Check sheet for the drawn part. Datum: minimum x, y, z corner. Units: mm. A direction names the side the tool comes from. Coordinates: 2 decimals unless noted, no trailing zeros. Loops run counter-clockwise (first coordinate to the right, second up) from the corner with the lowest first, then second, coordinate; pieces in that order, holes last.
Q1. Sectioned sample at A-A (z = 0.7). Count the separate pieces of the cut face and the enclosed holes in it, then the cut area to 3 significant figures.
Q2. Sectioned sample at C-C (y = 3). Enter the section's corners in (x, z), then the cut area to 3 significant figures.
Q3. Go/stop test with a flat-tipped pin: P1, Ø1, axis at x = 1.5, z = 5, coming from the -Y side. Record where the tip stops, or that it passes through.
Q4. Sectioned sample at D-D (y = 6.25). Enter the section's corners in (x, z).
Q5. Sectioned sample at B-B (x = 5). Enter the section's corners in (y, z).
Q6. Mould release check, pull along Z, two halves, no side actions. Record for the marked faces 3, 4 and 5: +Z half, -Z half, draft (parallel to the pull), parting line (faces both ways), or undercut.
Q7. Material ranges on probe 1 along Y at (x, z) = (5, 4.5); probe 2 along X at (y, z) = (7, 1.95); probe 3 along Y at (x, z) = (5, 0.6), recorded low to high.
Q8. Access from +Z, -Z, +X, -X, +Y, -Y to the whole of each face (thin tool, end or side, straight path). Record for the marked faces 1 and 2.
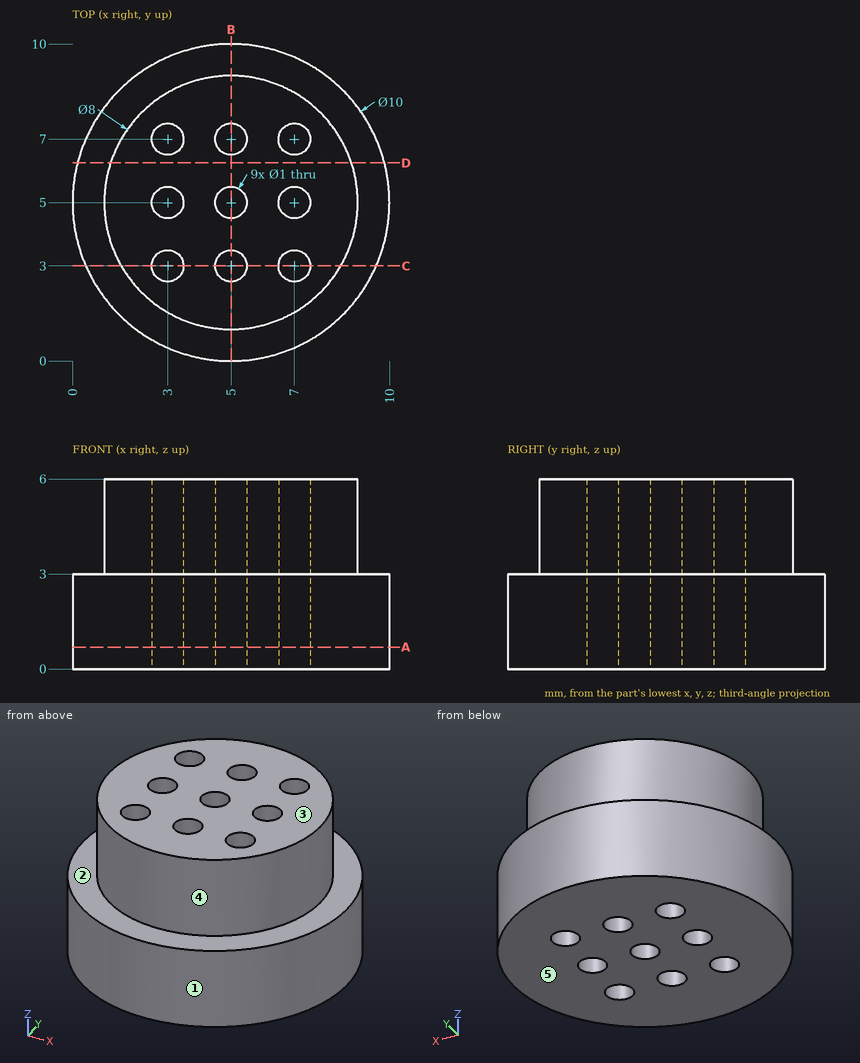
Geometry check:
1. separate pieces: 1
1. enclosed holes: 9
1. area: 71.5 mm2
2. outline: (0.42, 0) - (2.5, 0) - (2.5, 6) - (1.54, 6) - (1.54, 3) - (0.42, 3) - close; (3.5, 0) - (4.5, 0) - (4.5, 6) - (3.5, 6) - close; (5.5, 0) - (6.5, 0) - (6.5, 6) - (5.5, 6) - close; (7.5, 0) - (9.58, 0) - (9.58, 3) - (8.46, 3) - (8.46, 6) - (7.5, 6) - close
2. area: 30.3 mm2
3. P1: stops at y = 2.35
4. outline: (0.16, 0) - (9.84, 0) - (9.84, 3) - (8.8, 3) - (8.8, 6) - (1.2, 6) - (1.2, 3) - (0.16, 3) - close
5. outline: (0, 0) - (2.5, 0) - (2.5, 6) - (1, 6) - (1, 3) - (0, 3) - close; (3.5, 0) - (4.5, 0) - (4.5, 6) - (3.5, 6) - close; (5.5, 0) - (6.5, 0) - (6.5, 6) - (5.5, 6) - close; (7.5, 0) - (10, 0) - (10, 3) - (9, 3) - (9, 6) - (7.5, 6) - close
6. face 3: +Z half
6. face 4: draft
6. face 5: -Z half
7. probe 1: y = 1 to 2.5, 3.5 to 4.5, 5.5 to 6.5, 7.5 to 9
7. probe 2: x = 0.42 to 2.5, 3.5 to 4.5, 5.5 to 6.5, 7.5 to 9.58
7. probe 3: y = 0 to 2.5, 3.5 to 4.5, 5.5 to 6.5, 7.5 to 10
8. face 1: +Z, -Z
8. face 2: +Z
